Autodesk Inventor part; units mm, degrees
ref_plane "YZ Plane" through (0, 0, 0) normal (1, 0, 0) x (0, 1, 0)
ref_plane "XZ Plane" through (0, 0, 0) normal (0, 1, 0) x (-1, 0, 0)
ref_plane "XY Plane" through (0, 0, 0) normal (0, 0, 1) x (1, 0, 0)
sketch "Эскиз1" plane through (0, 0, 0) normal (0, 0, 1) x (1, 0, 0)
  line L0 (18.5, -18) -> (-18.5, -18)
  line L1 (-18.5, -18) -> (-18.5, 18)
  line L2 (-18.5, 18) -> (18.5, 18)
  line L3 (18.5, 18) -> (18.5, -18)
  line L4 (18.5, -18) -> (-18.5, 18) construction
  line L5 (-18.5, -18) -> (18.5, 18) construction
  line L6 (-14.5, -14.5) -> (14.5, -14.5) construction
  line L7 (14.5, -14.5) -> (14.5, 14.5) construction
  line L8 (14.5, 14.5) -> (-14.5, 14.5) construction
  line L9 (-14.5, 14.5) -> (-14.5, -14.5) construction
  line L10 (-14.5, -14.5) -> (14.5, 14.5) construction
  line L11 (14.5, -14.5) -> (-14.5, 14.5) construction
  circle A0 centre (-14.5, 14.5) radius 1.1
  circle A1 centre (14.5, 14.5) radius 1.1
  circle A2 centre (-14.5, -14.5) radius 1.1
  circle A3 centre (14.5, -14.5) radius 1.1
  point P0 (0, 0)
  dimension "d0" = 37
  dimension "d1" = 36
  dimension "d2" = 29
  dimension "d3" = 29
  dimension "d4" = 2.2
  dimension "d7" = 29
  dimension "d10" = 29
extrude "Выдавливание1" add sketch "Эскиз1" along normal blind 3
fillet "Сопряжение1" radius 1 4 edges at (-18.5, 18, 1.5) (18.5, 18, 1.5) (18.5, -18, 1.5) (-18.5, -18, 1.5)
sketch "Эскиз2" plane through (0, 0, 3) normal (0, 0, 1) x (1, 0, 0)
  circle A0 centre (10.5, -3.5) radius 1
  circle A1 centre (10.5, 10) radius 1
  circle A2 centre (-10.5, 10) radius 1
  circle A3 centre (-10.5, -3.5) radius 1
  point P0 (0, 0)
extrude "Выдавливание2" cut sketch "Эскиз2" against normal blind 3
sketch "Эскиз3" plane through (0, 0, 0) normal (0, 0, -1) x (-1, 0, 0)
  circle A0 centre (10.5, -3.5) radius 1
  circle A1 centre (-10.5, -3.5) radius 1
  circle A2 centre (10.5, 10) radius 1
  circle A3 centre (-10.5, 10) radius 1
  circle A4 centre (10.5, -3.5) radius 2
  circle A5 centre (-10.5, -3.5) radius 2
  circle A6 centre (-10.5, 10) radius 2
  circle A7 centre (10.5, 10) radius 2
  point P0 (0, 0)
  dimension "d18" = 1
  dimension "d19" = 1
  dimension "d20" = 1
  dimension "d21" = 1
extrude "Выдавливание3" cut sketch "Эскиз3" against normal blind 2
sketch "Эскиз4" plane through (0, 0, 3) normal (0, 0, 1) x (1, 0, 0)
  line L0 (-12.5, -12) -> (12.5, -12) construction
  line L1 (12.5, -12) -> (12.5, -18) construction
  line L2 (-17.5, -18) -> (17.5, -18) construction
  line L3 (-12.5, -12) -> (-12.5, -18) construction
  line L4 (12.5, -18) -> (-12.5, -18)
  line L5 (-12.5, -18) -> (-12.5, -11)
  line L6 (-12.5, -11) -> (12.5, -11)
  line L7 (12.5, -11) -> (12.5, -18)
  point P0 (0, 0)
  dimension "d24" = 7
extrude "Выдавливание4" cut sketch "Эскиз4" against normal blind 1
fillet "Сопряжение2" radius 0.5 9 edges at (0, -11, 3) (0, -11, 2) (0, -18, 2) (12.5, -18, 2.5) (12.5, -14.5, 2) (-12.5, -18, 2.5) (-12.5, -14.5, 2) (12.5, -14.5, 3) (-12.5, -14.5, 3)
properties part number "крепеж камеры"
Here's how the part is built. I have some questions about the finished solid (model axes, mm). A direction names the side the tool comes from. Round coordinates to 2 decimals unless told otherwise and drop trailing zeros. Order: outer loops, then holes, each group sorted by start corner. A loop starts at its lowest first (then second) coordinate and runs counter-clockwise, first axis right, second up. Notation, with made-up numbers: (46.5, -14) -> (74.5, -14) arc R13 cw to (74.5, 5) -> close; hole circle Ø10 at (71.25, 22). An arc over 180 degrees is marked (long way). Return JSON: item names as keys, results as strings.
Q1. Which directions (+Z, -Z, +X, -X, +Y, -Y) give clear straight access to the entire face, cutting with the end or side of a thin tool? Please do faces 1 (the cylindrical face through (11.974, 11.352, 0.986)), 2 (the cylindrical face through (18.199, -17.715, 1.521)).
Filled sheet:
{"face 1": "-Z", "face 2": "+Z, -Z, +X, -Y"}
Q2. If we section it at A-A on y = 10: List the corners of the cut face in (x, z) for me, plus the area to 3 significant figures.
Filled sheet:
{"outline": "(-18.5, 0) -> (-12.5, 0) -> (-12.5, 2) -> (-11.5, 2) -> (-11.5, 3) -> (-18.5, 3) -> close; (-9.5, 2) -> (-8.5, 2) -> (-8.5, 0) -> (8.5, 0) -> (8.5, 2) -> (9.5, 2) -> (9.5, 3) -> (-9.5, 3) -> close; (11.5, 2) -> (12.5, 2) -> (12.5, 0) -> (18.5, 0) -> (18.5, 3) -> (11.5, 3) -> close", "area": "91.0 mm^2"}
Q3. I need wall thicknesses on line 1 along X through (y, z) = (10, 2.7); line 2 along Y through (x, z) = (10.5, 2.3); line 3 along Y through (x, z) = (-15, 1.45). Which ranges of each line are inside material? Lowest first, please. Write a range as from..to.
Filled sheet:
{"line 1": "x = -18.5..-11.5, -9.5..9.5, 11.5..18.5", "line 2": "y = -11.04..-4.5, -2.5..9, 11..18", "line 3": "y = -18..-15.48, -13.52..13.52, 15.48..18"}
Q4. If we mould it in two halves opening along X, with no side actions, what happens to faces 3 (the flat face through (0, -14, 2)), 4 (the flat face through (0, 4, 3)), 5 (the flat face through (18.5, 0, 1))? For each: released by +X, released by -X, zero draft, split by the parting line, or undercut.
Filled sheet:
{"face 3": "undercut", "face 4": "zero draft", "face 5": "released by +X"}
Q5. If we section it at B-B on x = -10.5: Give the number of separate pieces and of enclosed holes in the cut face, plus the area to 3 significant figures.
Filled sheet:
{"separate pieces": "3", "enclosed holes": "0", "area": "80.9 mm^2"}
Q6. If we section it at D-D on y = 14.5: List the corners of the cut face in (x, z) for me.
Filled sheet:
{"outline": "(-18.5, 0) -> (-15.6, 0) -> (-15.6, 3) -> (-18.5, 3) -> close; (-13.4, 0) -> (13.4, 0) -> (13.4, 3) -> (-13.4, 3) -> close; (15.6, 0) -> (18.5, 0) -> (18.5, 3) -> (15.6, 3) -> close"}
Q7. For pin 1 Ø4.5 at (x, y) = (-11, 10.5) entering from -Z; pin 2 Ø6.5 at (x, y) = (-5, -15.5) entering from +Z, each with a flat end and sliding along its axis, tell me the tip position at first contact or that it passes through.
Filled sheet:
{"pin 1": "stops at z = 0", "pin 2": "stops at z = 2"}
